Model file for the job. Use its own axes, mm. A direction names the side the tool comes from. Coordinates: 2 decimals unless noted, no trailing zeros. Order: outer loops, then holes, each group sorted by start corner. A loop starts at its lowest first (then second) coordinate and runs counter-clockwise, first axis right, second up. Notation, with made-up numbers: (-19, 59) -> (13, 59) arc R15 cw to (13, 86) -> close; hole circle Ø2 at (49, 8.25). An arc over 180 degrees is marked (long way). Return JSON: item names as keys, results as strings. Group by question number.
1) Which spindle directions (+Z, -Z, +X, -X, +Y, -Y) get a long thin tool onto all of the face, cutting with end or side? Do faces 4 (the flat face through (1.2, -14.7, 0)), 5 (the flat face through (22, 0, 14)). Say none if no direction does.
2) Cut at D-D (y = -8.75). Write the cut outline in (x, z), and give its area (3 significant figures).
3) Pull direction Z, two halves, no side cores. Call faces 1 (the flat face through (-22, 0, 14)), 2 (the flat face through (-1, -16, 29.5)), 3 (the flat face through (-1.2, -14.7, 27.5)): +Z half, -Z half, draft (parallel to the pull), parting line (faces both ways), or undercut.
4) Probe line 1 (X direction, y = -12, z = 28); line 2 (X direction, y = -2.75, z = 18); line 3 (X direction, y = -24, z = 19). List the from-to ranges inside material, lowest first.
5) Cut at B-B (x = 0). Write the cut outline in (y, z), and give its area (4 significant figures).
6) Cut at C-C (z = 18). Write the cut outline in (x, y), and give its area (3 significant figures).
7) Flat gauge pins, fed straight in: pin 1 (12 mm diameter, centred on x = 7.5, z = 11.5, fed in from +Y); pin 2 (6 mm diameter, centred on y = -16.5, z = 19.5, fed in from -X); pin 3 (5 mm diameter, centred on y = -16, z = 11, fed in from -X). Where does each tip first touch, or does it go through?
8) Cut at A-A (y = -2.5). Write the cut outline in (x, z).
from build123d import *

# Parameters (mm, degrees)
BOSS_EXTRUDE1_DEPTH = 27.5
BOSS_EXTRUDE2_DEPTH = 2
BOSS_EXTRUDE3_DEPTH = 2


with BuildPart() as part:
    # Frame → Boss-Extrude1 (new body)
    with BuildSketch(Plane.XY):
        with BuildLine():
            Line((-45.033320997, -26), (45.033320997, -26))
            Line((45.033320997, -26), (30.022213998, 0))
            Line((30.022213998, 0), (18, 0))
            ThreePointArc((18, 0), (0, -18), (-18, 0))
            Line((-18, 0), (-30.022213998, 0))
            Line((-30.022213998, 0), (-45.033320997, -26))
        make_face()
        with BuildLine():
            ThreePointArc((-18, 0), (0, -18), (18, 0))
            Line((18, 0), (15, 0))
            ThreePointArc((15, 0), (0, -15), (-15, 0))
            Line((-15, 0), (-18, 0))
        make_face()
    extrude(amount=BOSS_EXTRUDE1_DEPTH)

    # lip → Boss-Extrude2 (add)
    with BuildSketch(Plane.XY.offset(27.5)):
        with BuildLine():
            Line((45.033320997, -26), (30.022213998, 0))
            Line((30.022213998, 0), (15, 0))
            ThreePointArc((15, 0), (0, -15), (-15, 0))
            Line((-15, 0), (-30.022213998, 0))
            Line((-30.022213998, 0), (-45.033320997, -26))
            Line((-45.033320997, -26), (45.033320997, -26))
        make_face()
        with BuildLine():
            ThreePointArc((14.5, 0), (0, -14.5), (-14.5, 0))
            Line((-14.5, 0), (-15, 0))
            ThreePointArc((-15, 0), (0, -15), (15, 0))
            Line((15, 0), (14.5, 0))
        make_face()
    extrude(amount=BOSS_EXTRUDE2_DEPTH)

    # lip2 → Boss-Extrude3 (add)
    with BuildSketch(Plane(origin=(0, 0, 0), x_dir=(-1, 0, 0), z_dir=(0, 0, -1))):
        with BuildLine():
            ThreePointArc((15, 0), (0, -15), (-15, 0))
            Line((-15, 0), (-30.022213998, 0))
            Line((-30.022213998, 0), (-45.033320997, -26))
            Line((-45.033320997, -26), (45.033320997, -26))
            Line((45.033320997, -26), (30.022213998, 0))
            Line((30.022213998, 0), (15, 0))
        make_face()
        with BuildLine():
            Line((-14.5, 0), (-15, 0))
            ThreePointArc((-15, 0), (0, -15), (15, 0))
            Line((15, 0), (14.5, 0))
            ThreePointArc((14.5, 0), (0, -14.5), (-14.5, 0))
        make_face()
    extrude(amount=BOSS_EXTRUDE3_DEPTH)


solid = part.part
Answers below:
{
 "1": {"face 4": "+Y", "face 5": "+Z, -Z, +X, -X, +Y"},
 "2": {"outline": "(-35.07, -2) -> (-11.56, -2) -> (-11.56, 0) -> (-12.18, 0) -> (-12.18, 27.5) -> (-11.56, 27.5) -> (-11.56, 29.5) -> (-35.07, 29.5) -> close; (11.56, -2) -> (35.07, -2) -> (35.07, 29.5) -> (11.56, 29.5) -> (11.56, 27.5) -> (12.18, 27.5) -> (12.18, 0) -> (11.56, 0) -> close", "area": "1,450 mm^2"},
 "3": {"face 1": "draft", "face 2": "+Z half", "face 3": "undercut"},
 "4": {"line 1": "x = -36.95 to -8.14, 8.14 to 36.95", "line 2": "x = -31.61 to -14.75, 14.75 to 31.61", "line 3": "x = -43.88 to 43.88"},
 "5": {"outline": "(-26, -2) -> (-14.5, -2) -> (-14.5, 0) -> (-15, 0) -> (-15, 27.5) -> (-14.5, 27.5) -> (-14.5, 29.5) -> (-26, 29.5) -> close", "area": "348.5 mm^2"},
 "6": {"outline": "(-45.03, -26) -> (45.03, -26) -> (30.02, 0) -> (15, 0) arc R15 cw to (-15, 0) -> (-30.02, 0) -> close", "area": "1,600 mm^2"},
 "7": {"pin 1": "stops at y = -6.54", "pin 2": "stops at x = -41.28", "pin 3": "stops at x = -40.7"},
 "8": {"outline": "(-31.47, -2) -> (-14.28, -2) -> (-14.28, 0) -> (-14.79, 0) -> (-14.79, 27.5) -> (-14.28, 27.5) -> (-14.28, 29.5) -> (-31.47, 29.5) -> close; (14.28, -2) -> (31.47, -2) -> (31.47, 29.5) -> (14.28, 29.5) -> (14.28, 27.5) -> (14.79, 27.5) -> (14.79, 0) -> (14.28, 0) -> close"}
}
